from build123d import *

# Parameters (mm, degrees)
SKETCH1_W                = 8.6
SKETCH1_H                = 8.7
SKETCH1_W_2              = 6.5
SKETCH1_H_2              = 5.9
BOSS_EXTRUDE1_DEPTH      = 24.7
SKETCH2_W                = 2
SKETCH2_H                = 1.51
BOSS_EXTRUDE2_DEPTH      = 1.95
BOSS_EXTRUDE2_DEPTH_BACK = 1.95
BOSS_EXTRUDE3_DEPTH      = 4.6
BOSS_EXTRUDE3_DEPTH_BACK = 4.6
CUT_EXTRUDE1_DEPTH       = 0.1


with BuildPart() as part:
    # Sketch1 → Boss-Extrude1 (new body)
    with BuildSketch(Plane.XY):
        Rectangle(SKETCH1_W, SKETCH1_H)
        Rectangle(SKETCH1_W_2, SKETCH1_H_2, mode=Mode.SUBTRACT)
    extrude(amount=BOSS_EXTRUDE1_DEPTH)

    # Sketch2 → Boss-Extrude2 (add, two sides)
    with BuildSketch(Plane.XY.offset(12.35)) as boss_extrude2_sk:
        with Locations((5.3, 3.595)):
            Rectangle(SKETCH2_W, SKETCH2_H)
        Polygon((4.3, 1.1), (5.63, 1.1), (5.63, -12.69), (8.2, -12.69), (8.2, -15.23), (6.2, -15.23), (4.3, -13.35), align=None)
    extrude(amount=BOSS_EXTRUDE2_DEPTH)
    extrude(boss_extrude2_sk.sketch, amount=-BOSS_EXTRUDE2_DEPTH_BACK)

    # Sketch3 → Boss-Extrude3 (add, two sides)
    with BuildSketch(Plane.XY.offset(12.35)) as boss_extrude3_sk:
        with BuildLine():
            Line((4.3, -4.35), (-4.3, -4.35))
            Line((-4.3, -4.35), (-4.3, -5.55))
            Line((-4.3, -5.55), (-1.15, -5.8))
            Line((-1.15, -5.8), (-1.15, -5.55))
            Line((-1.15, -5.55), (2.1, -5.55))
            Line((2.1, -5.55), (2.1, -6.75))
            Line((2.1, -6.75), (2.8, -6.75))
            ThreePointArc((2.8, -6.75), (3.365685425, -6.984314575), (3.6, -7.55))
            Line((3.6, -7.55), (3.6, -8.45))
            ThreePointArc((3.6, -8.45), (3.365685425, -9.015685425), (2.8, -9.25))
            Line((2.8, -9.25), (2.1, -9.25))
            Line((2.1, -9.25), (2.1, -10.45))
            Line((2.1, -10.45), (-1.15, -10.45))
            Line((-1.15, -10.45), (-1.15, -10.2))
            Line((-1.15, -10.2), (-4.3, -10.45))
            Line((-4.3, -10.45), (-4.3, -11.65))
            Line((-4.3, -11.65), (4.3, -11.65))
            Line((4.3, -11.65), (4.3, -4.35))
        make_face()
    extrude(amount=BOSS_EXTRUDE3_DEPTH)
    extrude(boss_extrude3_sk.sketch, amount=-BOSS_EXTRUDE3_DEPTH_BACK)

    # Sketch4 → Cut-Extrude1 (cut)
    with BuildSketch(Plane(origin=(0, 4.35, 0), x_dir=(1, 0, 0), z_dir=(0, 1, 0))):
        with BuildLine():
            Line((-0.16, -12.35), (-0.16, -16.85))
            Line((-0.16, -16.85), (-0.42, -16.85))
            ThreePointArc((-0.42, -16.85), (-0.773553391, -16.996446609), (-0.92, -17.35))
            Line((-0.92, -17.35), (-0.92, -20.05))
            ThreePointArc((-0.92, -20.05), (-0.773553391, -20.403553391), (-0.42, -20.55))
            Line((-0.42, -20.55), (2.8, -20.55))
            ThreePointArc((2.8, -20.55), (3.153553391, -20.403553391), (3.3, -20.05))
            Line((3.3, -20.05), (3.3, -17.35))
            ThreePointArc((3.3, -17.35), (3.153553391, -16.996446609), (2.8, -16.85))
            Line((2.8, -16.85), (2.54, -16.85))
            Line((2.54, -16.85), (2.54, -12.35))
            Line((2.54, -12.35), (2.54, -7.85))
            Line((2.54, -7.85), (2.8, -7.85))
            ThreePointArc((2.8, -7.85), (3.153553391, -7.703553391), (3.3, -7.35))
            Line((3.3, -7.35), (3.3, -4.65))
            ThreePointArc((3.3, -4.65), (3.153553391, -4.296446609), (2.8, -4.15))
            Line((2.8, -4.15), (-0.42, -4.15))
            ThreePointArc((-0.42, -4.15), (-0.773553391, -4.296446609), (-0.92, -4.65))
            Line((-0.92, -4.65), (-0.92, -7.35))
            ThreePointArc((-0.92, -7.35), (-0.773553391, -7.703553391), (-0.42, -7.85))
            Line((-0.42, -7.85), (-0.16, -7.85))
            Line((-0.16, -7.85), (-0.16, -12.35))
        make_face()
        with BuildLine():
            Line((2.34, -16.95), (2.34, -7.75))
            ThreePointArc((2.34, -7.75), (2.369289322, -7.679289322), (2.44, -7.65))
            Line((2.44, -7.65), (2.8, -7.65))
            ThreePointArc((2.8, -7.65), (3.012132034, -7.562132034), (3.1, -7.35))
            Line((3.1, -7.35), (3.1, -4.65))
            ThreePointArc((3.1, -4.65), (3.012132034, -4.437867966), (2.8, -4.35))
            Line((2.8, -4.35), (-0.42, -4.35))
            ThreePointArc((-0.42, -4.35), (-0.632132034, -4.437867966), (-0.72, -4.65))
            Line((-0.72, -4.65), (-0.72, -7.35))
            ThreePointArc((-0.72, -7.35), (-0.632132034, -7.562132034), (-0.42, -7.65))
            Line((-0.42, -7.65), (-0.06, -7.65))
            ThreePointArc((-0.06, -7.65), (0.010710678, -7.679289322), (0.04, -7.75))
            Line((0.04, -7.75), (0.04, -16.95))
            ThreePointArc((0.04, -16.95), (0.010710678, -17.020710678), (-0.06, -17.05))
            Line((-0.06, -17.05), (-0.42, -17.05))
            ThreePointArc((-0.42, -17.05), (-0.632132034, -17.137867966), (-0.72, -17.35))
            Line((-0.72, -17.35), (-0.72, -20.05))
            ThreePointArc((-0.72, -20.05), (-0.632132034, -20.262132034), (-0.42, -20.35))
            Line((-0.42, -20.35), (2.8, -20.35))
            ThreePointArc((2.8, -20.35), (3.012132034, -20.262132034), (3.1, -20.05))
            Line((3.1, -20.05), (3.1, -17.35))
            ThreePointArc((3.1, -17.35), (3.012132034, -17.137867966), (2.8, -17.05))
            Line((2.8, -17.05), (2.44, -17.05))
            ThreePointArc((2.44, -17.05), (2.369289322, -17.020710678), (2.34, -16.95))
        make_face(mode=Mode.SUBTRACT)
    extrude(amount=-CUT_EXTRUDE1_DEPTH, mode=Mode.SUBTRACT)


solid = part.part
Source: CAD feature listing. Evaluate the final solid. Frame: model axes, mm. A direction names the side the tool comes from. Round coordinates to 2 decimals unless told otherwise and drop trailing zeros. Loops run counter-clockwise (first coordinate to the right, second up) from the corner with the lowest first, then second, coordinate; pieces in that order, holes last. Notation, with made-up numbers: M 74.5,-32 L 122.5,-32 A19 ccw 122.5,-4 Z; hole C 2,-22.5 d1. An arc over 180 degrees is marked long. Answer as CSV lines item,"result".
Q1. Line query: line 1 along Y through (x, z) = (1, 17); line 2 along X through (y, z) = (2.75, 11.25); line 3 along X through (y, z) = (-3.75, 5.5). Output: solid intervals per line, ascending.
Verdict:
line 1,"y = -4.35 to -2.95, 2.95 to 4.35"
line 2,"x = -4.3 to -3.25, 3.25 to 4.3"
line 3,"x = -4.3 to 4.3"
Q2. Cut plane B-B (x = 5.25). Return the cut outline in (y, z).
Verdict:
outline,"M -14.29,10.4 L 1.1,10.4 L 1.1,14.3 L -14.29,14.3 Z; M 2.84,10.4 L 4.35,10.4 L 4.35,14.3 L 2.84,14.3 Z"
Q3. Cut plane C-C (z = 21.25). Return the cut outline in (x, y).
Verdict:
outline,"M -4.3,-4.35 L 4.3,-4.35 L 4.3,4.35 L -4.3,4.35 Z; hole M -3.25,-2.95 L 3.25,-2.95 L 3.25,2.95 L -3.25,2.95 Z"
Q4. Cut plane A-A (y = -1). Return the cut outline in (x, z).
Verdict:
outline,"M -4.3,0 L -3.25,0 L -3.25,24.7 L -4.3,24.7 Z; M 3.25,0 L 4.3,0 L 4.3,10.4 L 5.63,10.4 L 5.63,14.3 L 4.3,14.3 L 4.3,24.7 L 3.25,24.7 Z"
Q5. Reachability of faces 4 (the face through (0, -4.35, 21)), 5 (the face through (3.6, -8, 12)), 6 (the face through (5.63, -6, 12)) from +Z, -Z, +X, -X, +Y, -Y: full face, straight path, thin tool, end or side. Return the list, or none.
Verdict:
face 4,"+Z, +X, -X, -Y"
face 5,"+Z, -Z, -X"
face 6,"+Z, -Z, +X"
Q6. Contact query for flat-ended pins moving along their axis: pin 1 (0.5 mm diameter, centred on x = 5.5, y = 3.5, fed in from +Z); pin 2 (2.5 mm diameter, centred on x = 1, z = 11.5, fed in from -Y); pin 3 (6 mm diameter, centred on x = 6, y = -11, fed in from +Z); pin 4 (3 mm diameter, centred on y = -7, z = 20, fed in from +X). Output: stop coordinate, or through.
Verdict:
pin 1,"stops at z = 14.3"
pin 2,"stops at y = -11.65"
pin 3,"stops at z = 16.95"
pin 4,"passes through"
Q7. Pull-direction query (Y, two-part tool) for faces 1 (the face through (-4.3, -1, 13)), 2 (the face through (7, -15.23, 12)), 3 (the face through (-3.25, 0, 12)); classes: +Y half, -Y half, draft (parallel to the pull), parting line (faces both ways), or undercut.
Verdict:
face 1,"draft"
face 2,"-Y half"
face 3,"undercut"
Q8. Cut plane D-D (y = 1.75). Return the cut outline in (x, z).
Verdict:
outline,"M -4.3,0 L -3.25,0 L -3.25,24.7 L -4.3,24.7 Z; M 3.25,0 L 4.3,0 L 4.3,24.7 L 3.25,24.7 Z"
